The figure shows three views and two pictorial views of one solid part (mm, origin at its lowest corner). Answer the questions. A direction names the side the tool comes from. Round coordinates to 2 decimals unless told otherwise and drop trailing zeros. Write each loop counter-clockwise with the first axis right and the second up, starting at its lowest first coordinate (ties: lowest second). Pieces come first, ordered by that corner, then holes. Notation, with made-up numbers: M 85,-37.5 L 120,-37.5 A8 ccw 120,-27.5 Z; hole C 36,51.5 d6. An arc over 180 degrees is marked long. Answer in a Markdown table with one row per item.
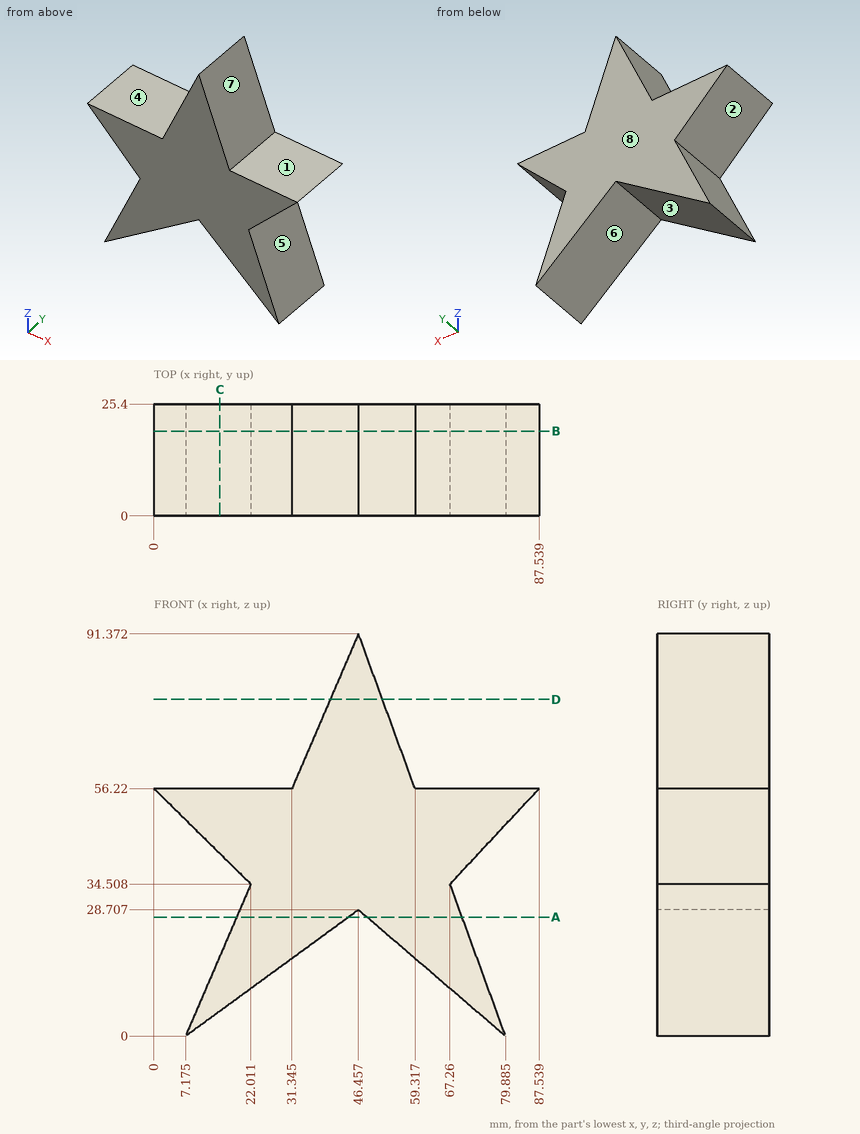
1. The part is cut by section A-A (z = 27). Determine the outline of the cut face in (x, y) (1 decimal).
Calculated:
| item | result |
|---|---|
| outline | M 18.8,0 L 44.1,0 L 44.1,25.4 L 18.8,25.4 Z; M 48.4,0 L 70,0 L 70,25.4 L 48.4,25.4 Z |
2. The part is cut by section B-B (y = 19.25). Determine the outline of the cut face in (x, z) (1 decimal).
Calculated:
| item | result |
|---|---|
| outline | M 0,56.2 L 22,34.5 L 7.2,0 L 46.5,28.7 L 79.9,0 L 67.3,34.5 L 87.5,56.2 L 59.3,56.2 L 46.5,91.4 L 31.3,56.2 Z |
3. Given pin 1 (3 mm diameter, centred on y = 18.5, z = 23.5, fed in from -X); pin 2 (5 mm diameter, centred on y = 9.5, z = 39, fed in from -X); pin 3 (8 mm diameter, centred on y = 20, z = 15, fed in from -X) (1 decimal), each flat-ended and moving along its own axis, determine where each tip first touches the part or whether it passes through.
Calculated:
| item | result |
|---|---|
| pin 1 | stops at x = 16.63 |
| pin 2 | stops at x = 14.92 |
| pin 3 | stops at x = 11.9 |
4. The part is cut by section C-C (x = 15). Determine the outline of the cut face in (y, z).
Calculated:
| item | result |
|---|---|
| outline | M 0,5.72 L 25.4,5.72 L 25.4,18.2 L 0,18.2 Z; M 0,41.42 L 25.4,41.42 L 25.4,56.22 L 0,56.22 Z |
5. A tool of negligible diameter and unlimited length cuts with its end or side. For the marked faces 1, 2, 3 and 4, from which of +Z, -Z, +X, -X, +Y, -Y can it reach the whole face along a straight path? Write none if from no direction.
Calculated:
| item | result |
|---|---|
| face 1 | +Z, +X, +Y, -Y |
| face 2 | -X, +Y, -Y |
| face 3 | -Z, +Y, -Y |
| face 4 | +Z, -X, +Y, -Y |
6. Determine the mould class of the marked faces 5, 6, 7 and 8 for opening direction Z: released by +Z, released by -Z, zero draft, split by the parting line, or undercut.
Calculated:
| item | result |
|---|---|
| face 5 | undercut |
| face 6 | released by -Z |
| face 7 | released by +Z |
| face 8 | zero draft |
7. Consider line 1 along X through (y, z) = (3.5, 18.5) (1 decimal); line 2 along Z through (x, y) = (14, 16) (1 decimal); line 3 along X through (y, z) = (10, 18) (1 decimal). Determine where each line is inside the solid, lowest interval first. Write a range as from..to.
Calculated:
| item | result |
|---|---|
| line 1 | x = 15.1..32.5, 58.3..73.1 |
| line 2 | z = 5..15.9, 42.4..56.2 |
| line 3 | x = 14.9..31.8, 58.9..73.3 |
8. The part is cut by section D-D (z = 76.5). Determine the outline of the cut face in (x, y).
Calculated:
| item | result |
|---|---|
| outline | M 40.06,0 L 51.9,0 L 51.9,25.4 L 40.06,25.4 Z |
